from build123d import *

# Parameters (mm, degrees)
EXTRUDE_1_DEPTH = 7.6
SHELL_1_T       = -0.3
SKETCH_2_W      = 0.2
SKETCH_2_H      = 1
EXTRUDE_2_DEPTH = 0.12
SKETCH_3_R      = 0.15
EXTRUDE_3_DEPTH = 4
FILLET_2_R      = 0.1


with BuildPart() as part:
    # 草图1 → 凸台-拉伸1 (new body)
    with BuildSketch(Plane(origin=(0, 0, 0), x_dir=(0, 0, -1), z_dir=(1, 0, 0))):
        Polygon((0, 0), (5.1, 0), (5.1, 5.5), (0, 5.5), (0, 5), (0.85, 5), (0.85, 4.15), (0, 4.15), align=None)
    extrude(amount=EXTRUDE_1_DEPTH)

    # 抽壳1
    shell_1_openings = [part.faces().sort_by_distance(p)[0] for p in [
        (3.8, 2.75, -5.1),
    ]]
    offset(amount=SHELL_1_T, openings=shell_1_openings, kind=Kind.INTERSECTION)

    # 草图2 → 凸台-拉伸2 (add)
    with BuildSketch(Plane.XZ):
        with Locations((2.8, -5.4)):
            Rectangle(SKETCH_2_W, SKETCH_2_H)
        with Locations((1.8, -5.4)):
            Rectangle(SKETCH_2_W, SKETCH_2_H)
        with Locations((3.8, -5.4)):
            Rectangle(SKETCH_2_W, SKETCH_2_H)
        with Locations((4.8, -5.4)):
            Rectangle(SKETCH_2_W, SKETCH_2_H)
        with Locations((5.8, -5.4)):
            Rectangle(SKETCH_2_W, SKETCH_2_H)
        with Locations((5.8, 0.3)):
            Rectangle(SKETCH_2_W, SKETCH_2_H)
        with Locations((4.8, 0.3)):
            Rectangle(SKETCH_2_W, SKETCH_2_H)
        with Locations((3.8, 0.3)):
            Rectangle(SKETCH_2_W, SKETCH_2_H)
        with Locations((2.8, 0.3)):
            Rectangle(SKETCH_2_W, SKETCH_2_H)
        with Locations((1.8, 0.3)):
            Rectangle(SKETCH_2_W, SKETCH_2_H)
    extrude(amount=EXTRUDE_2_DEPTH)

    # 草图3 → 凸台-拉伸3 (add)
    with BuildSketch(Plane(origin=(0, 0, -0.3), x_dir=(-1, 0, 0), z_dir=(0, 0, -1))):
        with Locations((-5.8, 1.4)):
            Circle(SKETCH_3_R)
        with Locations((-4.8, 1.4)):
            Circle(SKETCH_3_R)
        with Locations((-3.8, 1.4)):
            Circle(SKETCH_3_R)
        with Locations((-2.8, 1.4)):
            Circle(SKETCH_3_R)
        with Locations((-1.8, 1.4)):
            Circle(SKETCH_3_R)
        with Locations((-1.8, 2.8)):
            Circle(SKETCH_3_R)
        with Locations((-2.8, 2.8)):
            Circle(SKETCH_3_R)
        with Locations((-3.8, 2.8)):
            Circle(SKETCH_3_R)
        with Locations((-4.8, 2.8)):
            Circle(SKETCH_3_R)
        with Locations((-5.8, 2.8)):
            Circle(SKETCH_3_R)
    extrude(amount=EXTRUDE_3_DEPTH)

    # 圆角2
    fillet_2_edges = [part.edges().sort_by_distance(p)[0] for p in [
        (0, 5.5, -2.55),
        (0, 2.75, -5.1),
        (0, 2.075, 0),
        (7.6, 2.75, -5.1),
        (3.8, 4.15, 0),
        (3.8, 5, 0),
        (3.8, 5.5, 0),
        (7.6, 5.5, -2.55),
        (7.6, 5.25, 0),
        (7.6, 5, -0.425),
        (7.6, 4.575, -0.85),
        (7.6, 4.15, -0.425),
        (7.6, 2.075, 0),
        (0, 4.15, -0.425),
        (7.6, 0, -2.55),
        (0, 4.575, -0.85),
        (0, 5, -0.425),
        (0, 5.25, 0),
    ]]
    fillet(fillet_2_edges, radius=FILLET_2_R)


solid = part.part
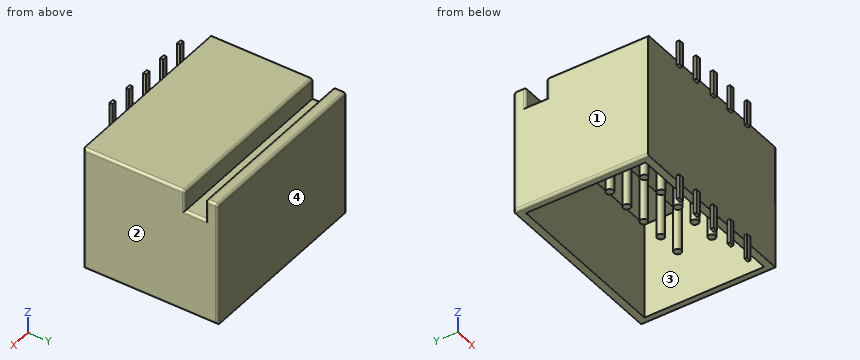
Verification items for the finished model (mm, model axes). Face numbers are marked on the shaded views. Coordinates: 2 decimals unless noted, no trailing zeros. Order: outer loops, then holes, each group sorted by start corner. A loop starts at its lowest first (then second) coordinate and runs counter-clockwise, first axis right, second up.
1. Sectioned sample at C-C, the plane y = 4.35. Record the cut outline in (x, z).
Results found:
outline: (0, -5) arc R0.1 ccw to (0.1, -5.1) - (0.3, -5.1) - (0.3, -1.15) - (7.3, -1.15) - (7.3, -5.1) - (7.5, -5.1) arc R0.1 ccw to (7.6, -5) - (7.6, -0.95) arc R0.1 ccw to (7.5, -0.85) - (0.1, -0.85) arc R0.1 ccw to (0, -0.95) - close
2. Go/stop test with flat-tipped pins: pin 1 Ø2 at (x, y) = (1.5, 2) entering from +Z; pin 2 Ø0.8 at (x, z) = (3.5, -0.5) entering from -Y; pin 3 Ø0.7 at (x, y) = (5.5, 4.5) entering from -Z; pin 4 Ø1.5 at (x, z) = (1.5, -1.5) entering from -Y. Record where each tip stops, or that it passes through.
Results found:
pin 1: stops at z = 0
pin 2: stops at y = -0.12
pin 3: stops at z = -1.15
pin 4: stops at y = 0
3. Release check for a two-part mould opening along X. For the marked faces 1, 2, 3 and 4 record: +X half, -X half, draft (parallel to the pull), parting line (faces both ways), or undercut.
Results found:
face 1: -X half
face 2: +X half
face 3: undercut
face 4: draft
4. Scan lines: line 1 (Y direction, x = 3.5, z = -0.75); line 2 (Y direction, x = 1, z = -3.75); line 3 (X direction, y = 2.15, z = -3). Record each from-to range of solid material in increasing order.
Results found:
line 1: y = 0 to 0.3, 3.85 to 4.15, 5 to 5.5
line 2: y = 0 to 0.3, 5.2 to 5.5
line 3: x = 0 to 0.3, 7.3 to 7.6
5. Sectioned sample at A-A, the plane z = -2.25. Give the number of separate pieces and of enclosed holes in the cut face, and give its area (3 significant figures).
Results found:
separate pieces: 11
enclosed holes: 1
area: 8.20 mm2
6. Sectioned sample at D-D, the plane z = -4.75. Record the cut outline in (x, y), and give its area (3 significant figures).
Results found:
outline: (0, 0) - (7.5, 0) arc R0.1 ccw to (7.6, 0.1) - (7.6, 5.4) arc R0.1 ccw to (7.5, 5.5) - (0.1, 5.5) arc R0.1 ccw to (0, 5.4) - close; hole (0.3, 0.3) - (7.3, 0.3) - (7.3, 5.2) - (0.3, 5.2) - close
area: 7.49 mm2
